from build123d import *

# Parameters (mm, degrees)
SKETCH1_W           = 48
SKETCH1_H           = 25
BOSS_EXTRUDE1_DEPTH = 4
SKETCH2_W           = 30
SKETCH2_H           = 25
BOSS_EXTRUDE2_DEPTH = 10
SKETCH3_R           = 1.5
CUT_EXTRUDE1_DEPTH  = 15
SKETCH4_R           = 1.6
CUT_EXTRUDE2_DEPTH  = 15


with BuildPart() as part:
    # Sketch1 → Boss-Extrude1 (new body)
    with BuildSketch(Plane(origin=(0, 0, 0), x_dir=(1, 0, 0), z_dir=(0, 1, 0))):
        Rectangle(SKETCH1_W, SKETCH1_H)
    extrude(amount=BOSS_EXTRUDE1_DEPTH)

    # Sketch2 → Boss-Extrude2 (add)
    with BuildSketch(Plane(origin=(0, 4, 0), x_dir=(1, 0, 0), z_dir=(0, 1, 0))):
        Rectangle(SKETCH2_W, SKETCH2_H)
    extrude(amount=BOSS_EXTRUDE2_DEPTH)

    # Sketch3 → Cut-Extrude1 (cut, through all)
    with BuildSketch(Plane(origin=(0, 14, 0), x_dir=(1, 0, 0), z_dir=(0, 1, 0))):
        with Locations(Location((0, 7.975, 0), (0, 0, 270))):  # turned: the seam where the file's is
            Circle(SKETCH3_R)
        with Locations(Location((0, -7.975, 0), (0, 0, 270))):  # turned: the seam where the file's is
            Circle(SKETCH3_R)
        with Locations(Location((-11, 7.5, 0), (0, 0, 270))):  # turned: the seam where the file's is
            Circle(SKETCH3_R)
        with Locations(Location((-11, -7.5, 0), (0, 0, 270))):  # turned: the seam where the file's is
            Circle(SKETCH3_R)
    extrude(amount=-CUT_EXTRUDE1_DEPTH, mode=Mode.SUBTRACT)

    # Sketch4 → Cut-Extrude2 (cut, through all)
    with BuildSketch(Plane.XZ):
        with Locations(Location((-20, 9, 0), (0, 0, 270))):  # turned: the seam where the file's is
            Circle(SKETCH4_R)
        with Locations(Location((20, 9, 0), (0, 0, 270))):  # turned: the seam where the file's is
            Circle(SKETCH4_R)
        with Locations(Location((20, -9, 0), (0, 0, 270))):  # turned: the seam where the file's is
            Circle(SKETCH4_R)
        with Locations(Location((-20, -9, 0), (0, 0, 270))):  # turned: the seam where the file's is
            Circle(SKETCH4_R)
    extrude(amount=-CUT_EXTRUDE2_DEPTH, mode=Mode.SUBTRACT)


solid = part.part
Input: part model. Units: mm. Frame: model coordinates. A direction names the side the tool comes from. Coordinates: 2 decimals unless noted, no trailing zeros. Order: outer loops, then holes, each group sorted by start corner. A loop starts at its lowest first (then second) coordinate and runs counter-clockwise, first axis right, second up. Notation, with made-up numbers: M 33.5,71.5 L 79.5,71.5 A17 ccw 79.5,100.5 Z; hole C -40,29 d9. An arc over 180 degrees is marked long. Write item = value, one per line. Start each with the question number.
(1) Reachability of faces 1 (the flat face through (-24, 2, 0)), 2 (the flat face through (-15, 9, 0)), 3 (the flat face through (15, 9, 0)) from +Z, -Z, +X, -X, +Y, -Y: full face, straight path, thin tool, end or side. Return the list, or none.
(2) Pull-direction query (Z, two-part tool) for faces 4 (the flat face through (19, 4, 0)), 5 (the cylindrical face through (-0.575, 7.098, 9.361)), 6 (the flat face through (0, 5, 12.5)); classes: released by +Z, released by -Z, zero draft, split by the parting line, or undercut.
(3) Section D-D on x = 0. Output: boundary loops of the cut face in (y, z) (3 decimals).
(4) First-contact query: P1, Ø4.5, axis at x = 18.5, z = -5.5, coming from the +Y side; P2, Ø1.8, axis at x = 0, z = -7.975, coming from the +Y side; P3, Ø3, axis at y = 9.5, z = 6, coming from the +X side; P4, Ø8, axis at y = 9, z = 1, coming from the -X side. Flat tips, straight axial feed; report the tip coordinate or a pass-through.
(5) Section B-B on y = 7.5. Output: boundary loops of the cut face in (x, z) (3 decimals), and give its area (3 significant figures).
(6) Section C-C on z = -8. Output: boundary loops of the cut face in (x, y), and give its area (3 significant figures).
(7) Line query: line 1 along X through (y, z) = (4.5, -7.5); line 2 along Z through (x, y) = (-19, 2.75); line 3 along Y through (x, z) = (-18, 2.75). Output: solid intervals per line, ascending. Write a range as [from, to].
(8) Section A-A on x = 20. Output: boundary loops of the cut face in (y, z).
Result set:
q1.face_1 = +Z, -Z, -X, +Y, -Y
q1.face_2 = +Z, -Z, -X, +Y
q1.face_3 = +Z, -Z, +X, +Y
q2.face_4 = zero draft
q2.face_5 = undercut
q2.face_6 = released by +Z
q3.outline = M 0,-12.5 L 14,-12.5 L 14,-9.475 L 0,-9.475 Z; M 0,-6.475 L 14,-6.475 L 14,6.475 L 0,6.475 Z; M 0,9.475 L 14,9.475 L 14,12.5 L 0,12.5 Z
q4.P1 = 4
q4.P2 = through
q4.P3 = 15
q4.P4 = -15
q5.outline = M -15,-12.5 L 15,-12.5 L 15,12.5 L -15,12.5 Z; hole C -11,-7.5 d3; hole C -11,7.5 d3; hole C 0,-7.975 d3; hole C 0,7.975 d3
q5.area = 722 mm²
q6.outline = M -24,0 L -21.25,0 L -21.25,4 L -24,4 Z; M -18.75,0 L -12.41,0 L -12.41,14 L -15,14 L -15,4 L -18.75,4 Z; M -9.59,0 L -1.5,0 L -1.5,14 L -9.59,14 Z; M 1.5,0 L 18.75,0 L 18.75,4 L 15,4 L 15,14 L 1.5,14 Z; M 21.25,0 L 24,0 L 24,4 L 21.25,4 Z
q6.area = 390 mm²
q7.line_1 = [-15, -12.5], [-9.5, -1.42], [1.42, 15]
q7.line_2 = [-12.5, -10.25], [-7.75, 7.75], [10.25, 12.5]
q7.line_3 = [0, 4]
q8.outline = M 0,-12.5 L 4,-12.5 L 4,-10.6 L 0,-10.6 Z; M 0,-7.4 L 4,-7.4 L 4,7.4 L 0,7.4 Z; M 0,10.6 L 4,10.6 L 4,12.5 L 0,12.5 Z
